Check sheet for the modelled part. Datum: model origin and axes. Units: mm. Round coordinates to 2 decimals unless told otherwise and drop trailing zeros. Loops run counter-clockwise (first coordinate to the right, second up) from the corner with the lowest first, then second, coordinate; pieces in that order, holes last. Notation, with made-up numbers: (-18.5, 42.25) -> (11.5, 42.25) arc R19 cw to (11.5, 71.25) -> close; hole circle Ø2 at (28, 63.5). An arc over 180 degrees is marked (long way). Use one line per item in the form item = value. Start each with the question number.
(1) Sectioned sample at B-B (x = -8). Record the cut outline in (y, z).
(2) Sectioned sample at C-C (z = 0). Record the cut outline in (x, y), and give its area (3 significant figures).
(3) Go/stop test with a flat-tipped pin: pin 1 (2.5 mm diameter, centred on x = 21.4, z = 21.4, fed in from +Y). Record where the tip stops, or that it passes through.
(4) Material ranges on probe 1 along Z at (x, y) = (-21.4, 1.8); probe 2 along Z at (x, y) = (10.7, 1.95); probe 3 along X at (y, z) = (1.7, -7), recorded low to high. Write a range as [from, to].
(5) Sectioned sample at A-A (z = -10.7). Record the cut outline in (x, y), and give its area (3 significant figures).
(6) Sectioned sample at D-D (y = 1.8). State how many separate pieces and enclosed holes the cut face has, and give its area (3 significant figures).
from build123d import *

# Parameters (mm, degrees)
SKETCH_1_W          = 54.8
SKETCH_1_H          = 54.8
SKETCH_1_R          = 4.1
SKETCH_1_R_2        = 1.6
EXTRUDE_1_DEPTH     = 4.4
FILLET_1_R          = 6
SKETCH_2_R          = 1.6
CUT_EXTRUDE_1_DEPTH = 10


with BuildPart() as part:
    # 草图1 → 凸台-拉伸1 (new body)
    with BuildSketch(Plane(origin=(0, 0, 0), x_dir=(1, 0, 0), z_dir=(0, 1, 0))):
        Rectangle(SKETCH_1_W, SKETCH_1_H)
        Circle(SKETCH_1_R, mode=Mode.SUBTRACT)
        with Locations((21.4, 21.4)):
            Circle(SKETCH_1_R_2, mode=Mode.SUBTRACT)
        with Locations((21.4, -21.4)):
            Circle(SKETCH_1_R_2, mode=Mode.SUBTRACT)
        with Locations((-21.4, -21.4)):
            Circle(SKETCH_1_R_2, mode=Mode.SUBTRACT)
        with Locations((-21.4, 21.4)):
            Circle(SKETCH_1_R_2, mode=Mode.SUBTRACT)
        Polygon((17.7, -5), (17.7, 5), (17.7, 10), (22.4, 10), (22.4, 5), (22.4, -5), (22.4, -10), (17.7, -10), align=None, mode=Mode.SUBTRACT)
        Polygon((-5, 17.7), (-10, 17.7), (-10, 22.4), (-5, 22.4), (5, 22.4), (10, 22.4), (10, 17.7), (5, 17.7), align=None, mode=Mode.SUBTRACT)
        Polygon((5, -17.7), (10, -17.7), (10, -22.4), (5, -22.4), (-5, -22.4), (-10, -22.4), (-10, -17.7), (-5, -17.7), align=None, mode=Mode.SUBTRACT)
        Polygon((-17.7, 5), (-17.7, -5), (-17.7, -10), (-22.4, -10), (-22.4, -5), (-22.4, 5), (-22.4, 10), (-17.7, 10), align=None, mode=Mode.SUBTRACT)
    extrude(amount=EXTRUDE_1_DEPTH)

    # 圆角1
    fillet_1_edges = [part.edges().sort_by_distance(p)[0] for p in [
        (27.4, 2.2, 27.4),
        (-27.4, 2.2, 27.4),
        (-27.4, 2.2, -27.4),
        (27.4, 2.2, -27.4),
    ]]
    fillet(fillet_1_edges, radius=FILLET_1_R)

    # 草图2 → 切除-拉伸1 (cut)
    with BuildSketch(Plane(origin=(0, 4.4, 0), x_dir=(1, 0, 0), z_dir=(0, 1, 0))):
        with Locations((10.7, 10.7)):
            Circle(SKETCH_2_R)
        with Locations((10.7, -10.7)):
            Circle(SKETCH_2_R)
        with Locations((-10.7, -10.7)):
            Circle(SKETCH_2_R)
        with Locations((-10.7, 10.7)):
            Circle(SKETCH_2_R)
    extrude(amount=-CUT_EXTRUDE_1_DEPTH, mode=Mode.SUBTRACT)


solid = part.part
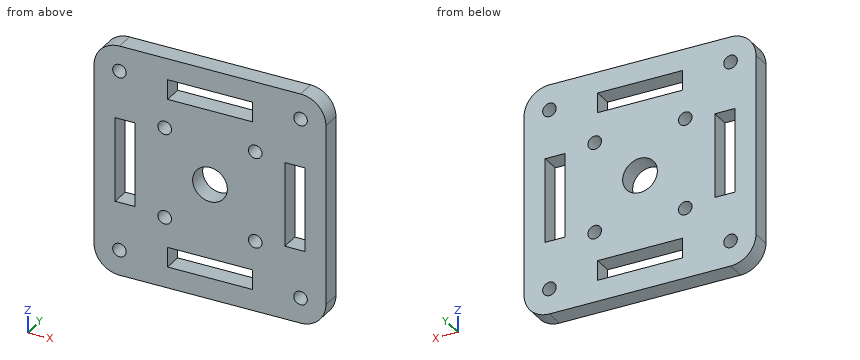
Checks:
q1.outline = (0, -27.4) -> (4.4, -27.4) -> (4.4, -22.4) -> (0, -22.4) -> close; (0, -17.7) -> (4.4, -17.7) -> (4.4, 17.7) -> (0, 17.7) -> close; (0, 22.4) -> (4.4, 22.4) -> (4.4, 27.4) -> (0, 27.4) -> close
q2.outline = (-27.4, 0) -> (-22.4, 0) -> (-22.4, 4.4) -> (-27.4, 4.4) -> close; (-17.7, 0) -> (-4.1, 0) -> (-4.1, 4.4) -> (-17.7, 4.4) -> close; (4.1, 0) -> (17.7, 0) -> (17.7, 4.4) -> (4.1, 4.4) -> close; (22.4, 0) -> (27.4, 0) -> (27.4, 4.4) -> (22.4, 4.4) -> close
q2.area = 164 mm2
q3.pin_1 = through
q4.probe_1 = [-27.4, -23], [-19.8, -10], [10, 19.8], [23, 27.4]
q4.probe_2 = [-27.4, -12.3], [-9.1, 9.1], [12.3, 27.4]
q4.probe_3 = [-27.4, -22.4], [-17.7, 17.7], [22.4, 27.4]
q5.outline = (-27.4, 0) -> (-12.3, 0) -> (-12.3, 4.4) -> (-27.4, 4.4) -> close; (-9.1, 0) -> (9.1, 0) -> (9.1, 4.4) -> (-9.1, 4.4) -> close; (12.3, 0) -> (27.4, 0) -> (27.4, 4.4) -> (12.3, 4.4) -> close
q5.area = 213 mm2
q6.separate_pieces = 1
q6.enclosed_holes = 13
q6.area = 2,480 mm2
